Could you check a few things on this model? Use its own coordinates, in mm. A direction names the side the tool comes from. Give positions to 0.01 mm unless a question says otherwise; leave off trailing zeros. Order: outer loops, then holes, each group sorted by start corner. A loop starts at its lowest first (then second) coordinate and runs counter-clockwise, first axis right, second up. Notation, with made-up numbers: (87.5, 25.5) - (146.5, 25.5) arc R23 ccw to (146.5, 46.5) - close; hole circle Ø8 at (-21.5, 25.5). An arc over 180 degrees is marked (long way). One line per question, with ' | ' between items. Start each with the question number.
1. Imagine slicing it at A-A (x = 79). Please give me the cut outline in (y, z), and give its area (3 significant figures).
2. Which directions (+Z, -Z, +X, -X, +Y, -Y) give clear straight access to the entire face, cutting with the end or side of a thin tool? Please do faces 4 (the cylindrical face through (242.91, 3.13, 54.44)), 5 (the flat face through (26, 3, -62.897)).
3. Imagine slicing it at D-D (z = -126). Please give me the cut outline in (x, y).
4. If we mould it in two halves opening along X, with no side actions, what happens to faces 1 (the cylindrical face through (-48.537, 3.131, -166.536)), 2 (the flat face through (247.185, 3, -57)), 3 (the flat face through (114.041, 3, -13))? For each: released by +X, released by -X, zero draft, split by the parting line, or undercut.
5. I need wall thicknesses on probe 1 along Z at (x, y) = (232, 4); probe 2 along Z at (x, y) = (185, 4.5); probe 3 along X at (y, z) = (1.75, -107). Which ranges of each line are inside material? Lowest first, please. Write a range as from..to.
6. Imagine slicing it at B-B (z = -9.5). Please give me the cut outline in (x, y).
7. For P1, Ø6, axis at x = -37.81, z = 43.95, coming from the -Y side, with a flat end and sliding along its axis, tell me the tip position at first contact or that it passes through.
8. Imagine slicing it at C-C (x = 149). Please give me the cut outline in (y, z), and give its area (3 significant figures).
```python
from build123d import *

# Parameters (mm, degrees)
SKETCH1_R           = 4.85
BOSS_EXTRUDE1_DEPTH = 6.35
SKETCH2_W           = 58.3
SKETCH2_H           = 70.3
CUT_EXTRUDE1_DEPTH  = 6.35
CUT_EXTRUDE2_DEPTH  = 6.35


with BuildPart() as part:
    # Sketch1 → Boss-Extrude1 (new body)
    with BuildSketch(Plane(origin=(0, 0, 0), x_dir=(1, 0, 0), z_dir=(0, 1, 0))):
        with BuildLine():
            Line((-37.814650179, 171.04710305), (232.185349821, 171.04710305))
            ThreePointArc((232.185349821, 171.04710305), (242.791951539, 166.653704768), (247.185349821, 156.04710305))
            Line((247.185349821, 156.04710305), (247.185349821, -43.95289695))
            ThreePointArc((247.185349821, -43.95289695), (242.791951539, -54.559498668), (232.185349821, -58.95289695))
            Line((232.185349821, -58.95289695), (-37.814650179, -58.95289695))
            ThreePointArc((-37.814650179, -58.95289695), (-48.421251896, -54.559498668), (-52.814650179, -43.95289695))
            Line((-52.814650179, -43.95289695), (-52.814650179, 156.04710305))
            ThreePointArc((-52.814650179, 156.04710305), (-48.421251896, 166.653704768), (-37.814650179, 171.04710305))
        make_face()
        with Locations((-37.814650179, 156.04710305)):
            Circle(SKETCH1_R, mode=Mode.SUBTRACT)
        with Locations((232.185349821, 156.04710305)):
            Circle(SKETCH1_R, mode=Mode.SUBTRACT)
        with Locations((232.185349821, -43.95289695)):
            Circle(SKETCH1_R, mode=Mode.SUBTRACT)
        with Locations((-37.814650179, -43.95289695)):
            Circle(SKETCH1_R, mode=Mode.SUBTRACT)
    extrude(amount=BOSS_EXTRUDE1_DEPTH)

    # Sketch2 → Cut-Extrude1 (cut)
    with BuildSketch(Plane.XZ):
        with Locations((168.185349821, -26.04710305)):
            Rectangle(SKETCH2_W, SKETCH2_H)
        with Locations((26.185349821, -98.04710305)):
            Rectangle(SKETCH2_W, SKETCH2_H)
    extrude(amount=-CUT_EXTRUDE1_DEPTH, mode=Mode.SUBTRACT)

    # Sketch3 → Cut-Extrude2 (cut)
    with BuildSketch(Plane.XZ):
        with BuildLine():
            Line((17.107545151, -28.900683481), (104.041408607, -28.900683481))
            ThreePointArc((104.041408607, -28.900683481), (111.112476419, -25.971751293), (114.041408607, -18.900683481))
            Line((114.041408607, -18.900683481), (114.041408607, -5.971842988))
            ThreePointArc((114.041408607, -5.971842988), (111.112476419, 1.099224823), (104.041408607, 4.028157012))
            Line((104.041408607, 4.028157012), (17.107545151, 4.028157012))
            ThreePointArc((17.107545151, 4.028157012), (10.03647734, 1.099224823), (7.107545151, -5.971842988))
            Line((7.107545151, -5.971842988), (7.107545151, -18.900683481))
            ThreePointArc((7.107545151, -18.900683481), (10.03647734, -25.971751293), (17.107545151, -28.900683481))
        make_face()
        with BuildLine():
            Line((110.251233871, -120.745362711), (197.185097326, -120.745362711))
            ThreePointArc((197.185097326, -120.745362711), (204.256165138, -117.816430523), (207.185097326, -110.745362711))
            Line((207.185097326, -110.745362711), (207.185097326, -97.816522218))
            ThreePointArc((207.185097326, -97.816522218), (204.256165138, -90.745454407), (197.185097326, -87.816522218))
            Line((197.185097326, -87.816522218), (110.251233871, -87.816522218))
            ThreePointArc((110.251233871, -87.816522218), (103.180166059, -90.745454407), (100.251233871, -97.816522218))
            Line((100.251233871, -97.816522218), (100.251233871, -110.745362711))
            ThreePointArc((100.251233871, -110.745362711), (103.180166059, -117.816430523), (110.251233871, -120.745362711))
        make_face()
    extrude(amount=-CUT_EXTRUDE2_DEPTH, mode=Mode.SUBTRACT)


solid = part.part
```
Results found:
1) outline: (0, -171.05) - (6.35, -171.05) - (6.35, -28.9) - (0, -28.9) - close; (0, 4.03) - (6.35, 4.03) - (6.35, 58.95) - (0, 58.95) - close | area: 1,250 mm2
2) face 4: +Z, +X, +Y, -Y | face 5: +Y, -Y
3) outline: (-52.81, 0) - (-2.96, 0) - (-2.96, 6.35) - (-52.81, 6.35) - close; (55.34, 0) - (247.19, 0) - (247.19, 6.35) - (55.34, 6.35) - close
4) face 1: released by -X | face 2: released by +X | face 3: undercut
5) probe 1: z = -171.05..-160.89, -151.2..39.11, 48.8..58.95 | probe 2: z = -171.05..-120.75, -87.82..-61.2, 9.1..58.95 | probe 3: x = -52.81..-2.96, 55.34..100.25, 207.19..247.19
6) outline: (-52.81, 0) - (7.11, 0) - (7.11, 6.35) - (-52.81, 6.35) - close; (114.04, 0) - (139.04, 0) - (139.04, 6.35) - (114.04, 6.35) - close; (197.34, 0) - (247.19, 0) - (247.19, 6.35) - (197.34, 6.35) - close
7) P1: passes through
8) outline: (0, -171.05) - (6.35, -171.05) - (6.35, -120.75) - (0, -120.75) - close; (0, -87.82) - (6.35, -87.82) - (6.35, -61.2) - (0, -61.2) - close; (0, 9.1) - (6.35, 9.1) - (6.35, 58.95) - (0, 58.95) - close | area: 805 mm2
